Read the model definition and answer for the solid it produces. Units are mm, in the model's axes. Give positions to 0.01 mm unless a question says otherwise; leave off trailing zeros. Loops run counter-clockwise (first coordinate to the right, second up) from the corner with the lowest first, then second, coordinate; pieces in that order, holes last. Notation, with made-up numbers: (35.25, 79.25) -> (87.25, 79.25) arc R26 ccw to (87.25, 112.25) -> close; hole circle Ø7 at (74, 9). An arc over 180 degrees is marked (long way). Return JSON: item names as keys, results as strings. Group by question number.
from build123d import *

# Parameters (mm, degrees)
SKETCH_1_R      = 1.5
EXTRUDE_1_DEPTH = 2


with BuildPart() as part:
    # 草图1 → 凸台-拉伸1 (new body)
    with BuildSketch(Plane.XY):
        with BuildLine():
            Line((-12.91723747, 0), (12.91723747, 0))
            ThreePointArc((12.91723747, 0), (17.453878353, 2.073310619), (18.855230664, 6.860370167))
            Line((18.855230664, 6.860370167), (9.744693373, 69.738315612))
            ThreePointArc((9.744693373, 69.738315612), (7.73338956, 73.414586328), (3.806700178, 74.877945445))
            Line((3.806700178, 74.877945445), (0, 74.877945445))
            Line((0, 74.877945445), (-3.806700178, 74.877945445))
            ThreePointArc((-3.806700178, 74.877945445), (-7.73338956, 73.414586328), (-9.744693373, 69.738315612))
            Line((-9.744693373, 69.738315612), (-18.855230664, 6.860370167))
            ThreePointArc((-18.855230664, 6.860370167), (-17.453878353, 2.073310619), (-12.91723747, 0))
        make_face()
        with Locations((-3, 50)):
            Circle(SKETCH_1_R, mode=Mode.SUBTRACT)
        with Locations((3, 50)):
            Circle(SKETCH_1_R, mode=Mode.SUBTRACT)
    extrude(amount=EXTRUDE_1_DEPTH)


solid = part.part
1. Section D-D on y = 38.5 is taken. Determine the outline of the cut face in (x, z).
2. Determine the mould class of faces 1 (the cylindrical face through (17.406, 2.019, 0.986)), 2 (the cylindrical face through (-17.5, 2.13, 0.99)), 3 (the cylindrical face through (2.675, 48.536, 0.986)) for opening direction X: pulls with the +X half, pulls with the -X half, needs draft (parallel to the pull), parting line crosses it, or undercut.
3. Section B-B on z = 1.05 is taken. Determine the outline of the cut face in (x, y), then the cut area to 3 significant figures.
4. Section A-A on x = 3 is taken. Determine the outline of the cut face in (y, z).
5. Section C-C on y = 50 is taken. Determine the outline of the cut face in (x, z), then the cut area to 3 significant figures.
6. Straight lines are drawn through the part: line 1 (Y direction, x = -3, z = 0.9); line 2 (X direction, y = 50.5, z = 0.8); line 3 (Y direction, x = 2.5, z = 1.9). For each, find the intervals that lie inside material, in ascending order. Write a range as from..to.
Completed:
{
 "1": {"outline": "(-14.27, 0) -> (14.27, 0) -> (14.27, 2) -> (-14.27, 2) -> close"},
 "2": {"face 1": "pulls with the +X half", "face 2": "pulls with the -X half", "face 3": "undercut"},
 "3": {"outline": "(-18.86, 6.86) arc R6 ccw to (-12.92, 0) -> (12.92, 0) arc R6 ccw to (18.86, 6.86) -> (9.74, 69.74) arc R6 ccw to (3.81, 74.88) -> (-3.81, 74.88) arc R6 ccw to (-9.74, 69.74) -> close; hole circle Ø3 at (-3, 50); hole circle Ø3 at (3, 50)", "area": "2,110 mm²"},
 "4": {"outline": "(0, 0) -> (48.5, 0) -> (48.5, 2) -> (0, 2) -> close; (51.5, 0) -> (74.88, 0) -> (74.88, 2) -> (51.5, 2) -> close"},
 "5": {"outline": "(-12.6, 0) -> (-4.5, 0) -> (-4.5, 2) -> (-12.6, 2) -> close; (-1.5, 0) -> (1.5, 0) -> (1.5, 2) -> (-1.5, 2) -> close; (4.5, 0) -> (12.6, 0) -> (12.6, 2) -> (4.5, 2) -> close", "area": "38.4 mm²"},
 "6": {"line 1": "y = 0..48.5, 51.5..74.88", "line 2": "x = -12.53..-4.41, -1.59..1.59, 4.41..12.53", "line 3": "y = 0..48.59, 51.41..74.88"}
}
